Source: CAD feature listing. Evaluate the final solid. Frame: model axes, mm. Coordinates: 2 decimals unless noted, no trailing zeros. Order: outer loops, then holes, each group sorted by start corner. A loop starts at its lowest first (then second) coordinate and runs counter-clockwise, first axis right, second up.
Item 1: Section C-C on x = 0. Return the cut outline in (y, z) (3 decimals), then the cut area to 3 significant figures.
Item 2: Ray query, line 1 (X direction, y = 2, z = 48); line 2 (Z direction, x = 31, y = 2.5); line 3 (X direction, y = 0.75, z = 24). Return the intervals inside material, ascending.
Item 3: Contact query for flat-ended pins moving along their axis: P1, Ø10, axis at x = -45.5, z = 50.5, coming from the +Y side (3 decimals); P2, Ø1, axis at y = 1.5, z = 23.5, coming from the +X side; P3, Ø1, axis at x = -36, y = 2, coming from the +Z side; P4, Ø5, axis at x = -43, y = 3.5, coming from the -Z side. Output: stop coordinate, or through.
Item 4: Section B-B on y = 2.25. State how many separate pieces and enclosed holes the cut face has, then the cut area to 3 significant figures.
Item 5: Section D-D on x = -17. Return the cut outline in (y, z) (1 decimal).
Item 6: Section A-A on z = 0. Return the cut outline in (x, y) (3 decimals).
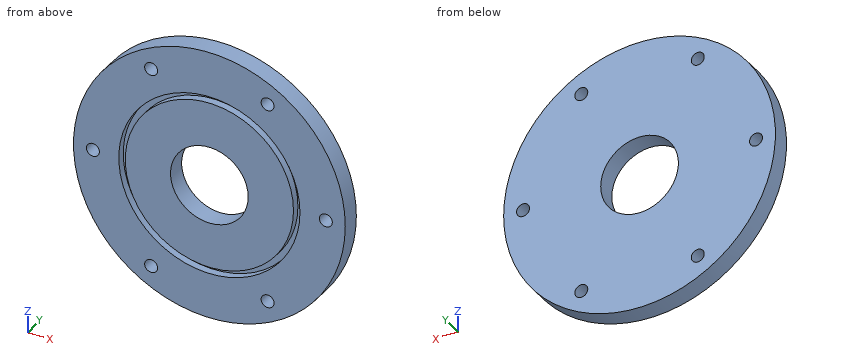
from build123d import *

# Parameters (mm, degrees)
SKETCH1_R                       = 66.675
SKETCH1_R_2                     = 19.05
BOSS_EXTRUDE1_DEPTH             = 9.525
SKETCH2_W                       = 3.175
SKETCH2_H                       = 3.81
F_1_4_0_25_DIAMETER_HOLE1_D     = 6.35
F_1_4_0_25_DIAMETER_HOLE1_DEPTH = 9.526
CIRPATTERN1_COUNT               = 6


with BuildPart() as part:
    # Sketch1 → Boss-Extrude1 (new body)
    with BuildSketch(Plane(origin=(0, 0, 0), x_dir=(1, 0, 0), z_dir=(0, 1, 0))):
        Circle(SKETCH1_R)
        Circle(SKETCH1_R_2, mode=Mode.SUBTRACT)
    extrude(amount=BOSS_EXTRUDE1_DEPTH)

    # Sketch2 → Cut-Revolve1 (revolve, cut)
    with BuildSketch(Plane.XY):
        with Locations((42.8625, 1.905)):
            Rectangle(SKETCH2_W, SKETCH2_H)
    revolve(axis=Axis((0, -0.47625, 0), (0, 1, 0)), mode=Mode.SUBTRACT)

    # 1/4 (0.25) Diameter Hole1
    with Locations(Plane(origin=(0, 9.525, 0), x_dir=(1, 0, 0), z_dir=(0, 1, 0))):
        with Locations((57.15, 0)):
            f_1_4_0_25_diameter_hole1 = Hole(F_1_4_0_25_DIAMETER_HOLE1_D / 2, depth=F_1_4_0_25_DIAMETER_HOLE1_DEPTH)

    # CirPattern1: 1/4 (0.25) Diameter Hole1 ×6 about axis
    cirpattern1_axis = Axis((0, 0, 0), (0, 1, 0))
    for i in range(1, CIRPATTERN1_COUNT):
        add(f_1_4_0_25_diameter_hole1.rotate(cirpattern1_axis, i * 360 / CIRPATTERN1_COUNT), mode=Mode.SUBTRACT)


solid = part.part
Answer list:
1. outline: (0, -66.675) - (9.525, -66.675) - (9.525, -19.05) - (0, -19.05) - (0, -41.275) - (3.81, -41.275) - (3.81, -44.45) - (0, -44.45) - close; (0, 19.05) - (9.525, 19.05) - (9.525, 66.675) - (0, 66.675) - (0, 44.45) - (3.81, 44.45) - (3.81, 41.275) - (0, 41.275) - close
1. area: 883 mm2
2. line 1: x = -46.28 to -31.38, -25.77 to 25.77, 31.38 to 46.28
2. line 2: z = -59.03 to -51.54, -47.44 to -31.86, -27.25 to 27.25, 31.86 to 47.44, 51.54 to 59.03
2. line 3: x = -62.21 to -37.41, -33.58 to 33.58, 37.41 to 62.21
3. P1: stops at y = 9.525
3. P2: stops at x = 62.58
3. P3: stops at z = 56.44
3. P4: stops at z = -52.97
4. separate pieces: 2
4. enclosed holes: 8
4. area: 11,800 mm2
5. outline: (0, -64.5) - (9.5, -64.5) - (9.5, -8.6) - (0, -8.6) - (0, -37.6) - (3.8, -37.6) - (3.8, -41.1) - (0, -41.1) - close; (0, 8.6) - (9.5, 8.6) - (9.5, 64.5) - (0, 64.5) - (0, 41.1) - (3.8, 41.1) - (3.8, 37.6) - (0, 37.6) - close
6. outline: (-66.675, 0) - (-60.325, 0) - (-60.325, 9.525) - (-66.675, 9.525) - close; (-53.975, 0) - (-44.45, 0) - (-44.45, 3.81) - (-41.275, 3.81) - (-41.275, 0) - (-19.05, 0) - (-19.05, 9.525) - (-53.975, 9.525) - close; (19.05, 0) - (41.275, 0) - (41.275, 3.81) - (44.45, 3.81) - (44.45, 0) - (53.975, 0) - (53.975, 9.525) - (19.05, 9.525) - close; (60.325, 0) - (66.675, 0) - (66.675, 9.525) - (60.325, 9.525) - close
